Part model, mm, in its own coordinate system. A direction names the side the tool comes from. Give positions to 0.01 mm unless a question says otherwise; leave off trailing zeros. Write each loop counter-clockwise with the first axis right and the second up, starting at its lowest first coordinate (ties: lowest second). Pieces come first, ordered by that corner, then holes. Notation, with made-up numbers: M -29,-33 L 27,-33 A25 ccw 27,-15 Z; hole C 69.5,-20.75 d8. An arc over 180 degrees is marked long. Use a Markdown table: item, result.
```python
from build123d import *

# Parameters (mm, degrees)
SKETCH1_W           = 103
SKETCH1_H           = 91.5
SKETCH1_R           = 2.15
SKETCH1_R_2         = 2.25
BOSS_EXTRUDE1_DEPTH = 23
SKETCH2_R           = 7.625
SKETCH2_R_2         = 6.875
BOSS_EXTRUDE2_DEPTH = 30.31
SKETCH4_R           = 4.9
BOSS_EXTRUDE3_DEPTH = 14.15
BOSS_EXTRUDE4_START = -133.31
SKETCH2_7_R         = 7.625
SKETCH2_7_R_2       = 6.875
BOSS_EXTRUDE4_DEPTH = 30.31
SKETCH6_W           = 41.6
SKETCH6_H           = 91.5
BOSS_EXTRUDE5_DEPTH = 15.3
SKETCH6_5_W         = 10.3
SKETCH6_5_H         = 91.5
BOSS_EXTRUDE7_DEPTH = 33


with BuildPart() as part:
    # Sketch1 → Boss-Extrude1 (new body)
    with BuildSketch(Plane(origin=(0, 0, 0), x_dir=(1, 0, 0), z_dir=(0, 1, 0))):
        Rectangle(SKETCH1_W, SKETCH1_H)
        with Locations(Location((-47, 28.1, 0), (0, 0, 270))):
            Circle(SKETCH1_R, mode=Mode.SUBTRACT)
        with Locations(Location((-47, 12.1, 0), (0, 0, 270))):
            Circle(SKETCH1_R, mode=Mode.SUBTRACT)
        with Locations(Location((47, 28.1, 0), (0, 0, 270))):
            Circle(SKETCH1_R_2, mode=Mode.SUBTRACT)
        with Locations(Location((47, 12.1, 0), (0, 0, 270))):
            Circle(SKETCH1_R_2, mode=Mode.SUBTRACT)
    extrude(amount=BOSS_EXTRUDE1_DEPTH)

    # Sketch2 → Boss-Extrude2 (add)
    with BuildSketch(Plane.ZY.offset(51.5)):
        with Locations((-35.95, 11.5)):
            Circle(SKETCH2_R)
        with Locations((-20.15, 15.2)):
            Circle(SKETCH2_R_2)
        with Locations((-4.25, 12.4)):
            Circle(SKETCH2_R)
    extrude(amount=BOSS_EXTRUDE2_DEPTH)

    # Sketch4 → Boss-Extrude3 (add)
    with BuildSketch(Plane(origin=(0, 0, -45.75), x_dir=(-1, 0, 0), z_dir=(0, 0, -1))):
        with Locations((5.8, 5.4)):
            Circle(SKETCH4_R)
        with Locations((0.8, 17.6)):
            Circle(SKETCH4_R)
        with Locations((11.3, 17.6)):
            Circle(SKETCH4_R)
        with Locations((16.3, 5.4)):
            Circle(SKETCH4_R)
        with Locations((21.8, 17.6)):
            Circle(SKETCH4_R)
        with Locations((26.8, 5.4)):
            Circle(SKETCH4_R)
        with Locations((32.3, 17.6)):
            Circle(SKETCH4_R)
        with Locations((37.3, 5.4)):
            Circle(SKETCH4_R)
    extrude(amount=BOSS_EXTRUDE3_DEPTH)

    # Sketch2<7> → Boss-Extrude4 (add)
    with BuildSketch(Plane.ZY.offset(51.5).offset(BOSS_EXTRUDE4_START)):
        with Locations((-35.95, 11.5)):
            Circle(SKETCH2_7_R)
        with Locations((-20.15, 15.2)):
            Circle(SKETCH2_7_R_2)
        with Locations((-4.25, 12.4)):
            Circle(SKETCH2_7_R)
    extrude(amount=BOSS_EXTRUDE4_DEPTH)

    # Sketch6 → Boss-Extrude5 (add)
    with BuildSketch(Plane(origin=(0, 23, 0), x_dir=(1, 0, 0), z_dir=(0, 1, 0))):
        with Locations((20.7, 0)):
            Rectangle(SKETCH6_W, SKETCH6_H)
    extrude(amount=BOSS_EXTRUDE5_DEPTH)

    # Sketch6<5> → Boss-Extrude7 (add)
    with BuildSketch(Plane(origin=(0, 23, 0), x_dir=(1, 0, 0), z_dir=(0, 1, 0))):
        with Locations((-17.05, 0)):
            Rectangle(SKETCH6_5_W, SKETCH6_5_H)
        with Locations((-6.25, 0)):
            Rectangle(SKETCH6_5_W, SKETCH6_5_H)
        with Locations((-27.85, 0)):
            Rectangle(SKETCH6_5_W, SKETCH6_5_H)
        with Locations((-38.65, 0)):
            Rectangle(SKETCH6_5_W, SKETCH6_5_H)
    extrude(amount=BOSS_EXTRUDE7_DEPTH)


solid = part.part
```
1. Two-plate mould, pull along X, no slides. Class faces 1 (the cylindrical face through (-31.326, 3.523, -52.726)), 2 (the flat face through (81.81, 12, -36)), 3 (the flat face through (-11, 18, -59.9)): released by +X, released by -X, zero draft, split by the parting line, or undercut.
Findings below:
| item | result |
|---|---|
| face 1 | undercut |
| face 2 | released by +X |
| face 3 | zero draft |
2. Drop flat-ended pins along their axis: P1, Ø3, axis at y = 43.5, z = 28, coming from the -X side; P2, Ø8, axis at x = 16, y = 12.5, coming from the -Z side; P3, Ø8, axis at x = 45, z = 22, coming from the +Y side. Give the stop position or say it passes through.
Findings below:
| item | result |
|---|---|
| P1 | x = -43.8 |
| P2 | z = -45.75 |
| P3 | y = 38.3 |
3. Tool access for faces 4 (the flat face through (-0.1, 31, 1)), 5 (the flat face through (46, 23, -1)), 6 (the flat face through (-48, 23, -1)): list every direction of +Z, -Z, +X, -X, +Y, -Y with a clear straight run to the whole face (end or side of a thin tool).
Findings below:
| item | result |
|---|---|
| face 4 | +Z, -Z, +Y |
| face 5 | +Z, -Z, +X, +Y |
| face 6 | +Z, -Z, -X, +Y |
4. Cut at B-B, the plane x = -47. Give the cut face in (y, z), then the cut area to 3 significant figures.
Findings below:
| item | result |
|---|---|
| outline | M 0,-45.75 L 23,-45.75 L 23,-30.25 L 0,-30.25 Z; M 0,-25.95 L 23,-25.95 L 23,-14.25 L 0,-14.25 Z; M 0,-9.95 L 23,-9.95 L 23,45.75 L 0,45.75 Z |
| area | 1,910 mm2 |
5. Drill centre lines: L1, parallel to X at y = 12, z = -12; L2, parallel to X at y = 42, z = 25.5; L3, parallel to X at y = 23.5, z = 10. Where is each one in solid material? Low to high.
Findings below:
| item | result |
|---|---|
| L1 | -51.5 to -49.15, -44.85 to 44.75, 49.25 to 51.5 |
| L2 | -43.8 to -33.5, -33 to -22.7, -22.2 to -11.9, -11.4 to -1.1 |
| L3 | -43.8 to -33.5, -33 to -22.7, -22.2 to -11.9, -11.4 to -1.1, -0.1 to 41.5 |
6. Cut at A-A, the plane y = 30. Give the cut face in (x, z), then the cut area to 3 significant figures.
Findings below:
| item | result |
|---|---|
| outline | M -43.8,-45.75 L -33.5,-45.75 L -33.5,45.75 L -43.8,45.75 Z; M -33,-45.75 L -22.7,-45.75 L -22.7,45.75 L -33,45.75 Z; M -22.2,-45.75 L -11.9,-45.75 L -11.9,45.75 L -22.2,45.75 Z; M -11.4,-45.75 L -1.1,-45.75 L -1.1,45.75 L -11.4,45.75 Z; M -0.1,-45.75 L 41.5,-45.75 L 41.5,45.75 L -0.1,45.75 Z |
| area | 7,580 mm2 |
7. Cut at C-C, the plane y = 41. Give the cut face in (x, z).
Findings below:
| item | result |
|---|---|
| outline | M -43.8,-45.75 L -33.5,-45.75 L -33.5,45.75 L -43.8,45.75 Z; M -33,-45.75 L -22.7,-45.75 L -22.7,45.75 L -33,45.75 Z; M -22.2,-45.75 L -11.9,-45.75 L -11.9,45.75 L -22.2,45.75 Z; M -11.4,-45.75 L -1.1,-45.75 L -1.1,45.75 L -11.4,45.75 Z |
8. Cut at D-D, the plane z = 6. Give the cut face in (x, y).
Findings below:
| item | result |
|---|---|
| outline | M -51.5,0 L 51.5,0 L 51.5,23 L 41.5,23 L 41.5,38.3 L -0.1,38.3 L -0.1,23 L -1.1,23 L -1.1,56 L -11.4,56 L -11.4,23 L -11.9,23 L -11.9,56 L -22.2,56 L -22.2,23 L -22.7,23 L -22.7,56 L -33,56 L -33,23 L -33.5,23 L -33.5,56 L -43.8,56 L -43.8,23 L -51.5,23 Z |
